```python
from build123d import *

# Parameters (mm, degrees)
SKETCH1_R           = 3.175
BOSS_EXTRUDE1_DEPTH = 6.35


with BuildPart() as part:
    # Sketch1 → Boss-Extrude1 (new body)
    with BuildSketch(Plane.XY):
        with BuildLine():
            Line((-81.15451448, 76.2), (95.90988075, 76.2))
            ThreePointArc((95.90988075, 76.2), (172.10988075, 0), (95.90988075, -76.2))
            Line((95.90988075, -76.2), (-81.15451448, -76.2))
            ThreePointArc((-81.15451448, -76.2), (-157.35451448, 0), (-81.15451448, 76.2))
        make_face()
        with Locations((8.184238886, 50.8)):
            Circle(SKETCH1_R, mode=Mode.SUBTRACT)
        with Locations((8.184238886, -50.8)):
            Circle(SKETCH1_R, mode=Mode.SUBTRACT)
        with Locations((-17.215761114, 50.8)):
            Circle(SKETCH1_R, mode=Mode.SUBTRACT)
        with Locations((33.584238886, 50.8)):
            Circle(SKETCH1_R, mode=Mode.SUBTRACT)
        with Locations((33.584238886, -50.8)):
            Circle(SKETCH1_R, mode=Mode.SUBTRACT)
        with Locations((-17.215761114, -50.8)):
            Circle(SKETCH1_R, mode=Mode.SUBTRACT)
        with Locations((7.377683135, 0)):
            Circle(SKETCH1_R, mode=Mode.SUBTRACT)
    extrude(amount=BOSS_EXTRUDE1_DEPTH)


solid = part.part
```
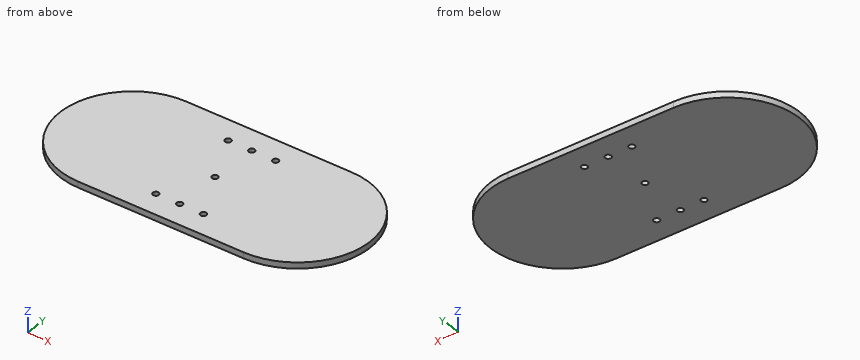
CAD build for the part. Positions are in the model's coordinates, mm. Coordinates: 2 decimals unless noted, no trailing zeros. Order: outer loops, then holes, each group sorted by start corner. A loop starts at its lowest first (then second) coordinate and runs counter-clockwise, first axis right, second up. Notation, with made-up numbers: (72.25, 73.5) - (80.25, 73.5) arc R18 ccw to (80.25, 86.5) - close; hole circle Ø6 at (-21.75, 17). An arc over 180 degrees is marked (long way). Use a Markdown table: item, result. Add a question column.
(1) Drill centre lines: line 1 along Y through (x, z) = (9, 4); line 2 along X through (y, z) = (-50.5, 5); line 3 along Y through (x, z) = (32, 4.5). Where is each one in solid material? Low to high. Write a range as [from, to].
(2) Saw through at B-B (z = 5). Give the cut face in (x, y) (3 decimals), then the cut area to 3 significant figures.
(3) Saw through at A-A (y = 0). Give the cut face in (x, z).
(4) Saw through at D-D (x = 124.5). Give the cut face in (y, z), then the cut area to 3 significant figures.
(5) Saw through at C-C (y = -50.8). Give the cut face in (x, z), then the cut area to 3 significant figures.
(6) Flat gauge pin, fed straight in: pin 1 (1 mm diameter, centred on y = 44, z = 5.5, fed in from -X). Where does the tip first touch, or does it go through?
Solved:
| question | item | result |
|---|---|---|
| 1 | line 1 | y = [-76.2, -53.87], [-47.73, -2.73], [2.73, 47.73], [53.87, 76.2] |
| 1 | line 2 | x = [-138.22, -20.38], [-14.05, 5.02], [11.35, 30.42], [36.75, 152.97] |
| 1 | line 3 | y = [-76.2, -53.55], [-48.05, 48.05], [53.55, 76.2] |
| 2 | outline | (-81.155, -76.2) - (95.91, -76.2) arc R76.2 ccw to (95.91, 76.2) - (-81.155, 76.2) arc R76.2 ccw to start; hole circle Ø6.35 at (-17.216, -50.8); hole circle Ø6.35 at (-17.216, 50.8); hole circle Ø6.35 at (7.378, 0); hole circle Ø6.35 at (8.184, -50.8); hole circle Ø6.35 at (8.184, 50.8); hole circle Ø6.35 at (33.584, -50.8); hole circle Ø6.35 at (33.584, 50.8) |
| 2 | area | 45,000 mm² |
| 3 | outline | (-157.35, 0) - (4.2, 0) - (4.2, 6.35) - (-157.35, 6.35) - close; (10.55, 0) - (172.11, 0) - (172.11, 6.35) - (10.55, 6.35) - close |
| 4 | outline | (-70.63, 0) - (70.63, 0) - (70.63, 6.35) - (-70.63, 6.35) - close |
| 4 | area | 897 mm² |
| 5 | outline | (-137.95, 0) - (-20.39, 0) - (-20.39, 6.35) - (-137.95, 6.35) - close; (-14.04, 0) - (5.01, 0) - (5.01, 6.35) - (-14.04, 6.35) - close; (11.36, 0) - (30.41, 0) - (30.41, 6.35) - (11.36, 6.35) - close; (36.76, 0) - (152.71, 0) - (152.71, 6.35) - (36.76, 6.35) - close |
| 5 | area | 1,720 mm² |
| 6 | pin 1 | stops at x = -143.72 |
